Design review of the part built by this model. Coordinates are the model's own, in mm. Face numbers are marked on the shaded views. Coordinates: 2 decimals unless noted, no trailing zeros. Loops run counter-clockwise (first coordinate to the right, second up) from the corner with the lowest first, then second, coordinate; pieces in that order, holes last. Notation, with made-up numbers: (12, 66.25) - (25, 66.25) arc R26 ccw to (25, 94.25) - close; hole circle Ø10 at (-17, 75). An arc over 180 degrees is marked (long way). Use one line per item in the form item = value. Start each with the question number.
(1) Add section D-D (z = 4.5). State the section outline as (x, y) points (3 decimals), plus the area to 3 significant figures.
(2) Add section C-C (x = 0.1). State the section outline as (y, z) points, plus the area to 3 significant figures.
(3) Add section B-B (y = 0). State the section outline as (x, z) points (3 decimals), plus the area to 3 significant figures.
(4) Clearance check with flat-ended pins moving along their axes: pin 1 Ø1.5 at (y, z) = (1, 5) entering from -X; pin 2 Ø2 at (x, z) = (-2.5, 2.5) entering from -Y; pin 3 Ø1.5 at (x, z) = (0, 5) entering from +Y (3 decimals); pin 4 Ø1.5 at (x, y) = (-1.5, 1) entering from +Z. State where each tip first meets the part, or that it passes through.
(5) For L1, parallel to Z at x = 2.35, y = -0.95; L2, parallel to Y at x = 0.1, z = 0.95; L3, parallel to Y at x = 0.4, z = 4.85, list the stretches that pass through material, from the lowest coordinate up.
(6) Add section A-A (x = -0.9). State the section outline as (y, z) points, plus the area to 3 significant figures.
(7) The part is to be moulded in two halves that separate along Z. For the marked faces 1, 2, 3 and 4, say which applies: pulls with the +Z half, pulls with the -Z half, needs draft (parallel to the pull), parting line crosses it, or undercut.
```python
from build123d import *

# Parameters (mm, degrees)
F0_R     = 0.725
F1_DEPTH = 6
F2_R     = 1.5
F3_DEPTH = 0.1
F4_R     = 3
F5_DEPTH = 0.5


with BuildPart() as f1:
    # F0 (on Top) → F1 (new body)
    with BuildSketch(Plane.XY):
        Circle(F0_R)
    extrude(amount=F1_DEPTH)

    # F2 (on face) → F3 (join)
    with BuildSketch(Plane.XY.offset(6)):
        Circle(F2_R)
    extrude(amount=-F3_DEPTH)

    # F4 (on face) → F5 (join)
    with BuildSketch(Plane(origin=(0, 0, 0), x_dir=(1, 0, 0), z_dir=(0, 0, -1))):
        Circle(F4_R)
    extrude(amount=-F5_DEPTH)


solid = f1.part
```
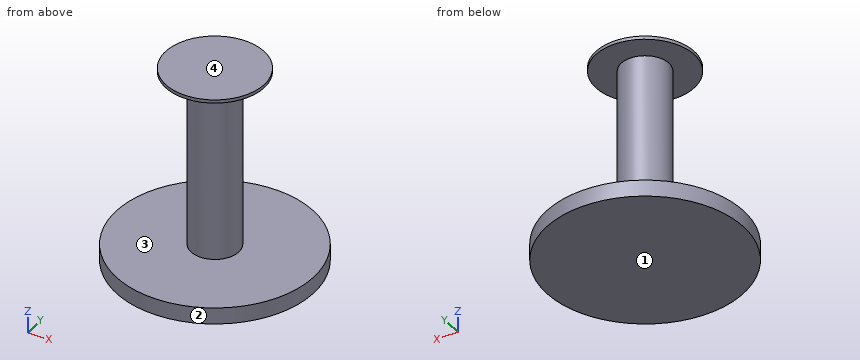
Computed values:
q1.outline = circle Ø1.45 at (0, 0)
q1.area = 1.65 mm^2
q2.outline = (-3, 0) - (3, 0) - (3, 0.5) - (0.72, 0.5) - (0.72, 5.9) - (1.5, 5.9) - (1.5, 6) - (-1.5, 6) - (-1.5, 5.9) - (-0.72, 5.9) - (-0.72, 0.5) - (-3, 0.5) - close
q2.area = 11.1 mm^2
q3.outline = (-3, 0) - (3, 0) - (3, 0.5) - (0.725, 0.5) - (0.725, 5.9) - (1.5, 5.9) - (1.5, 6) - (-1.5, 6) - (-1.5, 5.9) - (-0.725, 5.9) - (-0.725, 0.5) - (-3, 0.5) - close
q3.area = 11.1 mm^2
q4.pin_1 = -0.68
q4.pin_2 = through
q4.pin_3 = 0.725
q4.pin_4 = 6
q5.L1 = 0 to 0.5
q5.L2 = -0.72 to 0.72
q5.L3 = -0.6 to 0.6
q6.outline = (-2.86, 0) - (2.86, 0) - (2.86, 0.5) - (-2.86, 0.5) - close; (-1.2, 5.9) - (1.2, 5.9) - (1.2, 6) - (-1.2, 6) - close
q6.area = 3.10 mm^2
q7.face_1 = pulls with the -Z half
q7.face_2 = needs draft
q7.face_3 = undercut
q7.face_4 = pulls with the +Z half
